Autodesk Inventor part; units mm, degrees
ref_plane "YZ Plane" through (0, 0, 0) normal (1, 0, 0) x (0, 1, 0)
ref_plane "XZ Plane" through (0, 0, 0) normal (0, 1, 0) x (-1, 0, 0)
ref_plane "XY Plane" through (0, 0, 0) normal (0, 0, 1) x (1, 0, 0)
sketch "Sketch1" plane through (0, 0, 0) normal (0, 1, 0) x (-1, 0, 0)
  line L0 (-4, 0) -> (-36, 0)
  line L1 (-40, -4) -> (-40, -4)
  line L2 (-36, -8) -> (-4, -8)
  line L3 (0, -4) -> (0, -4)
  circle A0 centre (-36, -4) radius 2
  circle A1 centre (-4, -4) radius 2
  arc A2 (-4, -8) -> (0, -4) centre (-4, -4) ccw
  arc A3 (0, -4) -> (-4, 0) centre (-4, -4) ccw
  arc A4 (-36, 0) -> (-40, -4) centre (-36, -4) ccw
  arc A5 (-40, -4) -> (-36, -8) centre (-36, -4) ccw
  point P0 (0, 0)
  point P1 (-40, -8)
  point P2 (-40, 0)
  point P3 (0, -8)
  point P4 (-40, -4)
  point P5 (0, -4)
  dimension "d0" = 40
  dimension "d1" = 8
  dimension "d2" = 4
  dimension "d3" = 4
  dimension "d4" = 4
  dimension "d5" = 4
  dimension "d6" = 4
  dimension "d7" = 4
  dimension "d8" = 4
extrude "Extrusion1" add sketch "Sketch1" along normal blind 4
equation "\"d2\" = arm_rod_diam"
equation "\"d3\" = arm_rod_diam"
equation "\"d4\" = 0.5 * d1"
equation "\"d5\" = d4"
equation "\"d6\" = d4"
equation "\"d7\" = d5"
equation "\"d8\" = arm_rod_diam"
equation "\"arm_rod_diam\" = 4"
properties part number "config_arm"
Geometry: final body of the model. Coordinates: model frame, mm. Round coordinates to 2 decimals unless told otherwise and drop trailing zeros. Order: outer loops, then holes, each group sorted by start corner. A loop starts at its lowest first (then second) coordinate and runs counter-clockwise, first axis right, second up. Notation, with made-up numbers: M 83.5,39.25 L 88.5,39.25 A26 cw 88.5,60.25 Z; hole C 35,-30.75 d9. An arc over 180 degrees is marked long. Use one line per item in the form item = value. Start each with the question number.
Q1. Cut plane A-A (y = 2.3). Return loops of the section in (x, z).
Q2. Pin query (flat end, axial travel): pin 1 Ø2 at (y, z) = (2.5, -6.5) entering from -X. Return the tip coordinate at first contact, or that it passes through.
Q3. Cut plane B-B (z = -6.5). Return loops of the section in (x, y).
Q4. Material intervals for line 1 (Z direction, x = 36, y = 1.8); line 2 (X direction, y = 2, z = -4.5); line 3 (X direction, y = 1.15, z = -5.75), sorted ascending. Write a range as [from, to].
Q5. Mould query, pull axis Z, two halves, no side actions, for faces 1 (the face through (20, 2, -8)), 2 (the face through (40, 2, -4)), 3 (the face through (5.6, 2, -2.8)), 4 (the face through (20, 2, 0)). Classes: +Z half, -Z half, draft (parallel to the pull), parting line (faces both ways), or undercut.
Geometry results:
q1.outline = M 4,-8 L 36,-8 A4 ccw 36,0 L 4,0 A4 ccw Z; hole C 4,-4 d4; hole C 36,-4 d4
q2.pin_1 = 0.29
q3.outline = M 0.88,0 L 39.12,0 L 39.12,4 L 0.88,4 Z
q4.line_1 = [-8, -6], [-2, 0]
q4.line_2 = [0.03, 2.06], [5.94, 34.06], [37.94, 39.97]
q4.line_3 = [0.4, 3.03], [4.97, 35.03], [36.97, 39.6]
q5.face_1 = -Z half
q5.face_2 = parting line
q5.face_3 = undercut
q5.face_4 = +Z half
